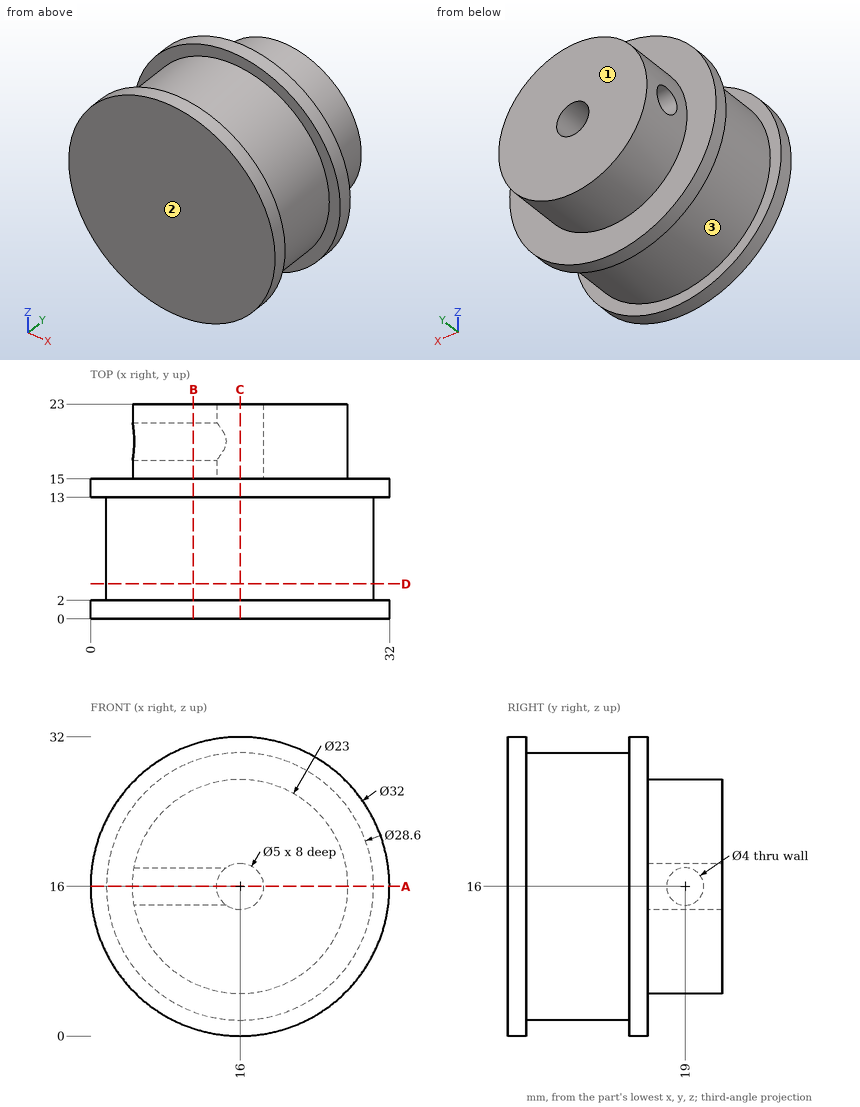
Study the drawing (mm; zero at the part's minimum x, y, z) and answer. Round coordinates to 2 decimals unless told otherwise and drop trailing zeros. Order: outer loops, then holes, each group sorted by start corner. A loop starts at its lowest first (then second) coordinate and runs counter-clockwise, first axis right, second up. Notation, with made-up numbers: (47, 59) - (93, 59) arc R17 ccw to (93, 92) - close; hole circle Ø4 at (-27.75, 80). An arc over 180 degrees is marked (long way). Use one line per item in the form item = value. Start each with the question number.
(1) Determine the mould class of the marked faces 1, 2 and 3 for opening direction Y: +Y half, -Y half, draft (parallel to the pull), parting line (faces both ways), or undercut.
(2) The part is cut by section A-A (z = 16). Give the vertices of the cut face in (x, y).
(3) Find the intervals of material crossed by line 1 along Y through (x, z) = (30.5, 20.5); line 2 along Y through (x, z) = (9.75, 16); line 3 along Y through (x, z) = (17.5, 15), in increasing order. Write a range as from..to.
(4) Flat-ended cylindrical pins translate along their axes: pin 1 Ø3 at (x, z) = (16, 16) entering from +Y; pin 2 Ø12 at (y, z) = (15, 24.5) entering from -X; pin 3 Ø2 at (x, y) = (5.5, 17) entering from +Z. Find the tip coordinate at first contact, or state that the pin passes through.
(5) The part is cut by section B-B (x = 11). Give the vertices of the cut face in (y, z).
(6) The part is cut by section C-C (x = 16). Give the vertices of the cut face in (y, z).
(7) The part is cut by section D-D (y = 3.75). Give the vertices of the cut face in (x, z), then the cut area to 3 significant figures.
Checked values:
q1.face_1 = +Y half
q1.face_2 = -Y half
q1.face_3 = undercut
q2.outline = (0, 0) - (32, 0) - (32, 2) - (30.3, 2) - (30.3, 13) - (32, 13) - (32, 15) - (27.5, 15) - (27.5, 23) - (18.5, 23) - (18.5, 15) - (13.5, 15) - (13.5, 17) - (4.5, 17) - (4.5, 15) - (0, 15) - (0, 13) - (1.7, 13) - (1.7, 2) - (0, 2) - close; (4.5, 21) - (13.5, 21) - (13.5, 23) - (4.5, 23) - close
q3.line_1 = 0..2, 13..15
q3.line_2 = 0..17, 21..23
q3.line_3 = 0..15
q4.pin_1 = 15
q4.pin_2 = 0.2
q4.pin_3 = 22.48
q5.outline = (0, 0.8) - (2, 0.8) - (2, 2.6) - (13, 2.6) - (13, 0.8) - (15, 0.8) - (15, 5.64) - (23, 5.64) - (23, 26.36) - (15, 26.36) - (15, 31.2) - (13, 31.2) - (13, 29.4) - (2, 29.4) - (2, 31.2) - (0, 31.2) - close; hole circle Ø4 at (19, 16)
q6.outline = (0, 0) - (2, 0) - (2, 1.7) - (13, 1.7) - (13, 0) - (15, 0) - (15, 4.5) - (23, 4.5) - (23, 13.5) - (15, 13.5) - (15, 18.5) - (23, 18.5) - (23, 27.5) - (15, 27.5) - (15, 32) - (13, 32) - (13, 30.3) - (2, 30.3) - (2, 32) - (0, 32) - close
q7.outline = circle Ø28.6 at (16, 16)
q7.area = 642 mm^2
